Autodesk Inventor part; units mm, degrees
ref_plane "YZ Plane" through (0, 0, 0) normal (1, 0, 0) x (0, 1, 0)
ref_plane "XZ Plane" through (0, 0, 0) normal (0, 1, 0) x (-1, 0, 0)
ref_plane "XY Plane" through (0, 0, 0) normal (0, 0, 1) x (1, 0, 0)
sketch "Sketch1" plane through (0, 0, 0) normal (0, 0, 1) x (1, 0, 0)
  line L0 (-102.5157, 69.2842) -> (97.4843, 69.2842)
  line L1 (97.4843, 69.2842) -> (97.4843, -80.7158)
  line L2 (97.4843, -80.7158) -> (-102.5157, -80.7158)
  line L3 (-102.5157, -80.7158) -> (-102.5157, 69.2842)
  point P0 (0, 0)
extrude "Extrusion1" add sketch "Sketch1" along normal blind 3
sketch "Sketch3" plane through (0, 0, 3) normal (0, 0, 1) x (1, 0, 0)
  point P0 (0, 0)
sketch "Sketch4" plane through (0, 0, 3) normal (0, 0, 1) x (1, 0, 0)
  line L0 (97.4843, 69.2842) -> (-102.5157, 69.2842)
  line L1 (-102.5157, 69.2842) -> (-99.5157, 69.2842)
  line L2 (-99.5157, 69.2842) -> (-99.5157, 19.2842)
  line L3 (-99.5157, 19.2842) -> (-102.5157, 19.2842)
  line L4 (-102.5157, 19.2842) -> (-102.5157, 69.2842)
  point P0 (0, 0)
extrude "Extrusion2" cut sketch "Sketch4" against normal blind 3
sketch "Sketch5" plane through (0, 0, 3) normal (0, 0, 1) x (1, 0, 0)
  line L0 (97.4843, -80.7158) -> (94.4843, -80.7158)
  line L1 (94.4843, -80.7158) -> (94.4843, -30.7158)
  line L2 (94.4843, -30.7158) -> (97.4843, -30.7158)
  line L3 (97.4843, -30.7158) -> (97.4843, -80.7158)
  point P0 (0, 0)
  point P1 (-102.5157, -80.7158)
  dimension "d17" = 3
  dimension "d18" = 50
extrude "Extrusion3" cut sketch "Sketch5" against normal blind 3
sketch "Sketch6" plane through (0, 0, 3) normal (0, 0, 1) x (1, 0, 0)
  line L0 (97.4843, -30.7158) -> (97.4843, 69.2842)
  line L1 (97.4843, 69.2842) -> (94.4843, 69.2842)
  line L2 (94.4843, 69.2842) -> (94.4843, 19.2842)
  line L3 (94.4843, 19.2842) -> (97.4843, 19.2842)
  line L4 (97.4843, 19.2842) -> (97.4843, 69.2842)
  point P0 (0, 0)
  dimension "d21" = 50
  dimension "d22" = 3
extrude "Extrusion4" cut sketch "Sketch6" against normal blind 3
sketch "Sketch7" plane through (0, 0, 3) normal (0, 0, 1) x (1, 0, 0)
  line L0 (-102.5157, 19.2842) -> (-102.5157, -80.7158)
  line L1 (-102.5157, -80.7158) -> (-99.5157, -80.7158)
  line L2 (-99.5157, -80.7158) -> (-99.5157, -30.7158)
  line L3 (-99.5157, -30.7158) -> (-102.5157, -30.7158)
  line L4 (-102.5157, -30.7158) -> (-102.5157, -80.7158)
  point P0 (0, 0)
  dimension "d25" = 50
  dimension "d26" = 3
extrude "Extrusion5" cut sketch "Sketch7" against normal blind 3
sketch "Sketch8" plane through (0, 0, 3) normal (0, 0, 1) x (1, 0, 0)
  line L0 (-102.5157, -30.7158) -> (-102.5157, 19.2842)
  line L1 (97.4843, -30.7158) -> (94.4843, -30.7158)
  line L2 (94.4843, -80.7158) -> (-99.5157, -80.7158)
  line L3 (-10.0157, -50.7158) -> (4.9843, -50.7158)
  line L4 (4.9843, -50.7158) -> (4.9843, -80.7158)
  line L5 (4.9843, -80.7158) -> (-10.0157, -80.7158)
  line L6 (-10.0157, -80.7158) -> (-10.0157, -50.7158)
  point P0 (0, 0)
  dimension "d32" = 15
  dimension "d33" = 30
extrude "Extrusion6" cut sketch "Sketch8" against normal blind 3
sketch "Sketch9" plane through (-10.0157, -80.7158, 3) normal (1, 0, 0) x (0, 0, -1)
  point P0 (3, 80.7158)
sketch "Sketch10" plane through (-10.0157, -50.7158, 3) normal (0, -1, 0) x (1, 0, 0)
  line L0 (15, 0) -> (15, -3)
  line L1 (15, -3) -> (0, -3)
  line L2 (15, 0) -> (0, 0)
  line L3 (0, 0) -> (0, -3)
  line L4 (0, -3) -> (15, -3)
  line L5 (15, -3) -> (15, 0)
  point P0 (10.0157, -3)
extrude "Extrusion7" add sketch "Sketch10" along normal blind 30
sketch "Sketch11" plane through (0, 0, 3) normal (0, 0, 1) x (1, 0, 0)
  line L0 (94.4843, -80.7158) -> (-99.5157, -80.7158)
  line L1 (-99.5157, -80.7158) -> (-99.5157, -30.7158)
  line L2 (97.4843, 19.2842) -> (97.4843, -30.7158)
  line L3 (-102.5157, -30.7158) -> (-102.5157, 19.2842)
  line L4 (-99.5157, 69.2842) -> (94.4843, 69.2842)
  point P0 (0, 0)
sketch "Sketch12" plane through (0, 0, 3) normal (0, 0, 1) x (1, 0, 0)
  circle A0 centre (34.4088, 18.4314) radius 1.5
  circle A1 centre (33.1388, -29.8286) radius 1.5
  circle A2 centre (-41.7912, -29.8286) radius 1.5
  circle A3 centre (-48.1412, 18.4314) radius 1.5
  point P0 (0, 0)
extrude "Extrusion8" cut sketch "Sketch12" against normal blind 3
sketch "Sketch13" plane through (0, 0, 3) normal (0, 0, 1) x (1, 0, 0)
  line L0 (-99.5157, 69.2842) -> (94.4843, 69.2842)
  line L1 (-102.5157, -30.7158) -> (-102.5157, 19.2842)
  line L2 (94.4843, -80.7158) -> (-99.5157, -80.7158)
  line L3 (-85.4157, 20.4542) -> (-70.4157, 20.4542)
  line L4 (-70.4157, 20.4542) -> (-70.4157, -31.8858)
  line L5 (-70.4157, -31.8858) -> (-85.4157, -31.8858)
  line L6 (-85.4157, -31.8858) -> (-85.4157, 20.4542)
  line L7 (-53.3157, 45.7842) -> (48.2843, 45.7842)
  line L8 (48.2843, 45.7842) -> (48.2843, 60.7842)
  line L9 (48.2843, 60.7842) -> (-53.3157, 60.7842)
  line L10 (-53.3157, 60.7842) -> (-53.3157, 45.7842)
  line L11 (65.3843, 20.4542) -> (80.3843, 20.4542)
  line L12 (80.3843, 20.4542) -> (80.3843, -31.8858)
  line L13 (80.3843, -31.8858) -> (65.3843, -31.8858)
  line L14 (65.3843, -31.8858) -> (65.3843, 20.4542)
  line L15 (97.4843, -30.7158) -> (97.4843, 19.2842)
  line L16 (94.4843, 69.2842) -> (94.4843, 19.2842)
  line L17 (-99.5157, 19.2842) -> (-99.5157, 69.2842)
  line L18 (-53.3157, -72.2158) -> (48.2843, -72.2158)
  line L19 (48.2843, -72.2158) -> (48.2843, -57.2158)
  line L20 (48.2843, -57.2158) -> (-53.3157, -57.2158)
  line L21 (-53.3157, -57.2158) -> (-53.3157, -72.2158)
  line L22 (-99.5157, -30.7158) -> (-99.5157, -80.7158)
  line L23 (94.4843, -30.7158) -> (94.4843, -80.7158)
  point P0 (0, 0)
extrude "Extrusion9" cut sketch "Sketch13" against normal blind 3
sketch "Sketch14" plane through (0, 0, 3) normal (0, 0, 1) x (1, 0, 0)
  circle A0 centre (-48.1412, 18.4314) radius 1.5
  circle A1 centre (-48.1412, 18.4314) radius 1.5
  circle A2 centre (34.4088, 18.4314) radius 1.5
  circle A3 centre (34.4088, 18.4314) radius 1.5
  circle A4 centre (33.1388, -29.8286) radius 1.5
  circle A5 centre (33.1388, -29.8286) radius 1.5
  circle A6 centre (-41.7912, -29.8286) radius 1.5
  circle A7 centre (-41.7912, -29.8286) radius 1.5
  point P0 (0, 0)
extrude "Extrusion10" add sketch "Sketch14" against normal blind 3
sketch "Sketch15" plane through (0, 0, 3) normal (0, 0, 1) x (1, 0, 0)
  point P0 (0, 0)
properties part number "Level2"
The model under review builds one solid part; all positions refer to its coordinate system, in mm. Round coordinates to 2 decimals unless told otherwise and drop trailing zeros. Write each loop counter-clockwise with the first axis right and the second up, starting at its lowest first coordinate (ties: lowest second). Pieces come first, ordered by that corner, then holes. Notation, with made-up numbers: M 40.25,9.5 L 67.25,9.5 A10 ccw 67.25,25.5 Z; hole C -16,16 d4. An arc over 180 degrees is marked long. Answer as CSV lines item,"result". Start each with the question number.
Q1. Consider section C-C, the plane z = 1.45. Give the boundary of the cut face in (x, y).
Q2. Wall thickness on line 1 along Y through (x, z) = (6, 2.3); line 2 along X through (y, z) = (-3.5, 1.4); line 3 along Y through (x, z) = (-73, 1.4): over which ranges is each line inside the solid? List them lowest first.
Q3. Consider section B-B, the plane x = -47. Give the boundary of the cut face in (y, z), then the cut area to 3 significant figures.
Q4. Consider section D-D, the plane x = -79.5. Give the boundary of the cut face in (y, z).
Q5. Clearance check with flat-ended pins moving along their axes: P1, Ø0.9, axis at y = -65.5, z = 2, coming from the -X side; P2, Ø0.9, axis at y = -57, z = 1, coming from the +X side. State where each tip first meets the part, or that it passes through.
Q6. Consider section A-A, the plane y = -68. Give the boundary of the cut face in (x, z).
Result set:
1,outline,"M -102.52,-30.72 L -99.52,-30.72 L -99.52,-80.72 L 94.48,-80.72 L 94.48,-30.72 L 97.48,-30.72 L 97.48,19.28 L 94.48,19.28 L 94.48,69.28 L -99.52,69.28 L -99.52,19.28 L -102.52,19.28 Z; hole M -85.42,-31.89 L -70.42,-31.89 L -70.42,20.45 L -85.42,20.45 Z; hole M -53.32,-72.22 L 48.28,-72.22 L 48.28,-57.22 L -53.32,-57.22 Z; hole M -53.32,45.78 L 48.28,45.78 L 48.28,60.78 L -53.32,60.78 Z; hole M 65.38,-31.89 L 80.38,-31.89 L 80.38,20.45 L 65.38,20.45 Z"
2,line 1,"y = -80.72 to -72.22, -57.22 to 45.78, 60.78 to 69.28"
2,line 2,"x = -102.52 to -85.42, -70.42 to 65.38, 80.38 to 97.48"
2,line 3,"y = -80.72 to -31.89, 20.45 to 69.28"
3,outline,"M -80.72,0 L -72.22,0 L -72.22,3 L -80.72,3 Z; M -57.22,0 L 45.78,0 L 45.78,3 L -57.22,3 Z; M 60.78,0 L 69.28,0 L 69.28,3 L 60.78,3 Z"
3,area,"360 mm²"
4,outline,"M -80.72,0 L -31.89,0 L -31.89,3 L -80.72,3 Z; M 20.45,0 L 69.28,0 L 69.28,3 L 20.45,3 Z"
5,P1,"stops at x = -99.52"
5,P2,"stops at x = 94.48"
6,outline,"M -99.52,0 L -53.32,0 L -53.32,3 L -99.52,3 Z; M 48.28,0 L 94.48,0 L 94.48,3 L 48.28,3 Z"
